Work out the finished part from the listing and answer in its coordinate system (mm). A direction names the side the tool comes from. Give positions to 0.01 mm unless a question says otherwise; leave off trailing zeros. Loops run counter-clockwise (first coordinate to the right, second up) from the corner with the lowest first, then second, coordinate; pieces in that order, holes last.
from build123d import *

# Parameters (mm, degrees)
SKETCH_W        = 29
SKETCH_H        = 47
PAD_DEPTH       = 40
SKETCH001_R     = 9.75
PAD001_DEPTH    = 10
SKETCH002_W     = 56
SKETCH002_H     = 6
POCKET_DEPTH    = 100
POCKET001_DEPTH = 5
SKETCH005_R     = 0.8
POCKET002_DEPTH = 5
SKETCH006_W     = 40
SKETCH006_H     = 20
PAD002_DEPTH    = 10
FILLET_R        = 9
FILLET001_R     = 9
SKETCH007_R     = 3
HOLE_DEPTH      = 50
SKETCH008_W     = 45
SKETCH008_H     = 54
POCKET003_DEPTH = 5
SKETCH009_W     = 40
SKETCH009_H     = 5
PAD003_DEPTH    = 50
PAD004_DEPTH    = 45
SKETCH011_W     = 40
SKETCH011_H     = 50
PAD005_DEPTH    = 50
POCKET004_DEPTH = 60.001
POCKET005_DEPTH = 40.001


with BuildPart() as part:
    # Sketch → Pad (new body)
    with BuildSketch(Plane.XY.offset(10)):
        with BuildLine():
            Line((0, 0), (40, 0))
            Line((40, 0), (40, 60))
            ThreePointArc((40, 60), (20, 68.990653), (0, 60))
            Line((0, 60), (0, 0))
        make_face()
        with Locations((20, 30)):
            Rectangle(SKETCH_W, SKETCH_H, mode=Mode.SUBTRACT)
    extrude(amount=PAD_DEPTH)

    # Sketch001 (on Face9 of Pad) → Pad001 (join)
    with BuildSketch(Plane(origin=(0, 0, 10), x_dir=(1, 0, 0), z_dir=(0, 0, -1))):
        with BuildLine():
            Line((40, -60), (40, 30))
            ThreePointArc((40, 30), (20, 50), (0, 30))
            Line((0, 30), (0, -60))
            ThreePointArc((0, -60), (20, -68.990653), (40, -60))
        make_face()
        with Locations((20, -42.25)):
            Circle(SKETCH001_R, mode=Mode.SUBTRACT)
    extrude(amount=PAD001_DEPTH)

    # Sketch002 (on Face7 of Pad001) → Pocket (cut)
    with BuildSketch(Plane(origin=(0, 0, 0), x_dir=(0, -1, 0), z_dir=(-1, 0, 0))):
        with Locations((-48, 3)):
            Rectangle(SKETCH002_W, SKETCH002_H)
    extrude(amount=-POCKET_DEPTH, mode=Mode.SUBTRACT)

    # Sketch003 (on Face4 of Pocket) → Pocket001 (cut)
    with BuildSketch(Plane.XY.offset(10)):
        with BuildLine():
            Line((0, 0), (40, 0))
            Line((40, 0), (40, -30))
            ThreePointArc((0, -30), (20, -50), (40, -30))
            Line((0, -30), (0, 0))
        make_face()
    extrude(amount=-POCKET001_DEPTH, mode=Mode.SUBTRACT)

    # Sketch005 → Pocket002 (cut)
    with BuildSketch(Plane(origin=(0, 0, 0), x_dir=(1, 0, 0), z_dir=(0, 0, -1))):
        with Locations((11.98, 30)):
            Circle(SKETCH005_R)
        with Locations((14.34, 35.7)):
            Circle(SKETCH005_R)
        with Locations((20, 37.98)):
            Circle(SKETCH005_R)
        with Locations((25.66, 35.7)):
            Circle(SKETCH005_R)
        with Locations((28.02, 30)):
            Circle(SKETCH005_R)
        with Locations((25.66, 24.35)):
            Circle(SKETCH005_R)
        with Locations((20, 22.02)):
            Circle(SKETCH005_R)
        with Locations((14.34, 24.34)):
            Circle(SKETCH005_R)
    extrude(amount=-POCKET002_DEPTH, mode=Mode.SUBTRACT)

    # Sketch006 (on Face17 of Pocket002) → Pad002 (join)
    with BuildSketch(Plane(origin=(0, 0, 0), x_dir=(1, 0, 0), z_dir=(0, 0, -1))):
        with Locations((20, -10)):
            Rectangle(SKETCH006_W, SKETCH006_H)
    extrude(amount=PAD002_DEPTH)

    # Fillet
    fillet_edges = [part.edges().sort_by_distance(p)[0] for p in [
        (20, 0, -10),
    ]]
    fillet(fillet_edges, radius=FILLET_R)

    # Fillet001
    fillet001_edges = [part.edges().sort_by_distance(p)[0] for p in [
        (20, 20, -10),
    ]]
    fillet(fillet001_edges, radius=FILLET001_R)

    # Sketch007 (on Face8 of Fillet001) → Hole (cut)
    with BuildSketch(Plane.YZ.offset(40)):
        with Locations((10, -5)):
            Circle(SKETCH007_R)
    extrude(amount=-HOLE_DEPTH, mode=Mode.SUBTRACT)

    # Sketch008 (on Face16 of Hole) → Pocket003 (cut)
    with BuildSketch(Plane.XY.offset(5)):
        with Locations((22.5, -27)):
            Rectangle(SKETCH008_W, SKETCH008_H)
    extrude(amount=-POCKET003_DEPTH, mode=Mode.SUBTRACT)

    # Sketch009 (on Face11 of Pocket003) → Pad003 (join)
    with BuildSketch(Plane.XZ):
        with Locations((20, 2.5)):
            Rectangle(SKETCH009_W, SKETCH009_H)
    extrude(amount=PAD003_DEPTH)

    # Sketch010 (on Face22 of Pad003) → Pad004 (join)
    with BuildSketch(Plane.XY.offset(5)):
        Polygon((0, 0), (0, -50), (40, -50), (40, 0), (35, 0), (35, -45), (5, -45), (5, 0), align=None)
    extrude(amount=PAD004_DEPTH)

    # Sketch011 (on Face22 of Pad004) → Pad005 (join)
    with BuildSketch(Plane.XZ.offset(50)):
        with Locations((20, 25)):
            Rectangle(SKETCH011_W, SKETCH011_H)
    extrude(amount=PAD005_DEPTH)

    # Sketch012 (on Face30 of Pad005) → Pocket004 (cut, through all)
    with BuildSketch(Plane.XY.offset(50)):
        Polygon((40, -50), (20, -92.890138), (0, -50), (0, -100), (40, -100), align=None)
    extrude(amount=-POCKET004_DEPTH, mode=Mode.SUBTRACT)

    # Sketch013 (on Face15 of Pocket004) → Pocket005 (cut, through all)
    with BuildSketch(Plane(origin=(0, 0, 0), x_dir=(0, -1, 0), z_dir=(-1, 0, 0))):
        Polygon((50, 0), (95, 0), (95, 50), (50, 50), (99.846928, 26.755996), (99.846928, 23.244004), align=None)
    extrude(amount=-POCKET005_DEPTH, mode=Mode.SUBTRACT)


solid = part.part
Item 1: Flat-ended cylindrical pins translate along their axes: pin 1 Ø1.5 at (y, z) = (-56, 28.5) entering from +X; pin 2 Ø23 at (x, z) = (15.5, 27.5) entering from -Y; pin 3 Ø5.5 at (x, z) = (23.5, 2.5) entering from +Y; pin 4 Ø10 at (x, y) = (5, -24) entering from -Z. Find the tip coordinate at first contact, or state that the pin passes through.
Item 2: Consider line 1 (X direction, y = -43, z = 44); line 2 (Z direction, x = 31, y = 10); line 3 (X direction, y = 17, z = 16). Determine where each line is inside the solid, lowest interval first.
Item 3: Find section C-C, the plane z = -3.5. Write down the section's boundary in (x, y), plus the area to 3 significant figures.
Item 4: For faces 4 (the face through (20, -45, 27)), 5 (the face through (20, 20, 3)), 6 (the face through (0, 6, 26)), determine the directions among +Z, -Z, +X, -X, +Y, -Y from which every point of the face is accessible in a straight line to the end or side of a thin tool.
Item 5: Find section D-D, the plane y = -1.5. Write down the section's boundary in (x, z).
Item 6: Determine the mould class of faces 1 (the face through (11, 50, 6)), 2 (the face through (20.28, 17.294, -7.434)), 3 (the face through (34.5, 30, 30)) for opening direction Y: released by +Y, released by -Y, zero draft, split by the parting line, or undercut.
Item 7: Find section A-A, the plane y = 42.25. Write down the section's boundary in (x, z).
Item 8: Find section B-B, the plane x = 3.5. Write down the section's boundary in (y, z).
Ans:
1. pin 1: stops at x = 37.55
1. pin 2: stops at y = -92.89
1. pin 3: stops at y = 20
1. pin 4: stops at z = 0
2. line 1: x = 0 to 5, 35 to 40
2. line 2: z = -10 to -8, -2 to 10
2. line 3: x = 0 to 5.5, 34.5 to 40
3. outline: (0, 0.35) - (40, 0.35) - (40, 7.4) - (0, 7.4) - close; (0, 12.6) - (40, 12.6) - (40, 19.65) - (0, 19.65) - close
3. area: 564 mm2
4. face 4: +Z
4. face 5: -Z, +X, -X, +Y
4. face 6: +Z, -Z, -X, +Y, -Y
5. outline: (0, 0) - (40, 0) - (40, 50) - (35, 50) - (35, 5) - (5, 5) - (5, 50) - (0, 50) - close
6. face 1: zero draft
6. face 2: released by +Y
6. face 3: undercut
7. outline: (0, 6) - (10.25, 6) - (10.25, 10) - (5.5, 10) - (5.5, 50) - (0, 50) - close; (29.75, 6) - (40, 6) - (40, 50) - (34.5, 50) - (34.5, 10) - (29.75, 10) - close
8. outline: (-57.51, 3.5) - (-50, 0) - (0, 0) - (0, -1) arc R9 ccw to (9, -10) - (11, -10) arc R9 ccw to (20, -1) - (20, 6) - (63.29, 6) - (63.29, 50) - (-50, 50) - (-57.51, 46.5) - close; hole circle Ø6 at (10, -5)
